from build123d import *

# Parameters (mm, degrees)
F0_W      = 95.881224
F0_H      = 68.022564
F0_R      = 16.769473
F1_DEPTH  = 25.4
F2_DEPTH  = 50.8
F4_DEPTH  = 25.4
F6_DEPTH  = 25.4
F8_DEPTH  = 0.254
F10_DEPTH = 0.0254


with BuildPart() as f1:
    # F0 (on Top) → F1 (new body)
    with BuildSketch(Plane.XY):
        Rectangle(F0_W, F0_H)
        Circle(F0_R, mode=Mode.SUBTRACT)
    extrude(amount=F1_DEPTH)

    # F0 (on Top) → F2 (join)
    with BuildSketch(Plane.XY):
        Circle(F0_R)
    extrude(amount=F2_DEPTH)

    # F3 (on Front) → F4 (cut)
    with BuildSketch(Plane.XZ):
        with BuildLine():
            ThreePointArc((16.7397, 50.897755), (-0.044019, 53.808078), (-16.71098, 50.290175))
            Line((-16.71098, 50.290175), (16.7397, 36.212575))
            Line((16.7397, 36.212575), (16.7397, 50.897755))
        make_face()
    extrude(amount=-F4_DEPTH, mode=Mode.SUBTRACT)

    # F5 (on Front) → F6 (cut)
    with BuildSketch(Plane.XZ):
        Polygon((-16.633531, 50.150838), (16.688788, 36.337622), (16.700679, 50.800726), (-16.633531, 50.828132), align=None)
    extrude(amount=F6_DEPTH, mode=Mode.SUBTRACT)

    # F7 (on Right) → F8 (cut)
    with BuildSketch(Plane.YZ):
        Polygon((-1.459569, 50.8672), (-1.681041, 36.348537), (0.976613, 36.348537), (0.976613, 50.8672), align=None)
    extrude(amount=F8_DEPTH, mode=Mode.SUBTRACT)

    # F9 (on Right) → F10 (cut)
    with BuildSketch(Plane.YZ):
        Polygon((-1.541382, 50.746284), (-1.648819, 36.371183), (0.972651, 36.371183), (0.972651, 50.746284), align=None)
    extrude(amount=-F10_DEPTH, mode=Mode.SUBTRACT)


solid = f1.part
Here's how the part is built. I have some questions about the finished solid (model axes, mm). A direction names the side the tool comes from. Round coordinates to 2 decimals unless told otherwise and drop trailing zeros. Loops run counter-clockwise (first coordinate to the right, second up) from the corner with the lowest first, then second, coordinate; pieces in that order, holes last. Notation, with made-up numbers: (33.25, 42) -> (67.25, 42) arc R7 cw to (67.25, 50) -> close; hole circle Ø4 at (79.25, 32.5). An arc over 180 degrees is marked (long way). Write each question's results on one line, items separated by ' | '.
(1) If we section it at C-C, the plane x = -26: List the corners of the cut face in (y, z) for me, then the cut area to 3 significant figures.
Worked answers:
outline: (-34.01, 0) -> (34.01, 0) -> (34.01, 25.4) -> (-34.01, 25.4) -> close | area: 1,730 mm2
(2) If we section it at A-A, the plane y = 5: List the corners of the cut face in (x, z) for me.
Worked answers:
outline: (-47.94, 0) -> (47.94, 0) -> (47.94, 25.4) -> (16.01, 25.4) -> (16.01, 36.52) -> (-16.01, 49.99) -> (-16.01, 25.4) -> (-47.94, 25.4) -> close; (-16.01, 50.58) arc R45.13 cw to (-15.44, 50.8) -> (-16.01, 50.8) -> close
(3) If we section it at B-B, the plane y = 21: List the corners of the cut face in (x, z) for me, then the cut area to 3 significant figures.
Worked answers:
outline: (-47.94, 0) -> (47.94, 0) -> (47.94, 25.4) -> (-47.94, 25.4) -> close | area: 2,440 mm2
(4) For faces 1 (the face through (-16.753, 0.737, 35.1)), 2 (the face through (-1, 0, 0)), 3 (the face through (-0.206, -6.404, 43.341)), which set-ups out of +Z, -Z, +X, -X, +Y, -Y let a thin tool reach every point of the face, with its end or its side?
Worked answers:
face 1: +Z | face 2: -Z, +X, -X, +Y, -Y | face 3: +Z, -Y
(5) For P1, Ø3, axis at y = -0.5, z = 40.5, coming from the +X side; P2, Ø0.5, axis at x = -16, z = 50.5, coming from the -Y side; P3, Ø20.5, axis at x = -3.5, y = 12.5, coming from the +Z side, each with a flat end and sliding along its axis, tell me the tip position at first contact or that it passes through.
Worked answers:
P1: x = 16.77 | P2: y = 0 | P3: z = 48.92
(6) We'd pull the mould along X, two halves only. Please class faces 4 (the face through (-11, 16, 25.4)), 5 (the face through (-0.22, 6.4, 43.35)), 6 (the face through (-47.941, 0, 13)), 7 (the face through (0.254, 0, 40)): released by +X, released by -X, zero draft, split by the parting line, or undercut.
Worked answers:
face 4: zero draft | face 5: undercut | face 6: released by -X | face 7: undercut
(7) If we section it at D-D, the plane z = 32.5: List the corners of the cut face in (x, y) for me, then the cut area to 3 significant figures.
Worked answers:
outline: circle Ø33.54 at (0, 0) | area: 883 mm2
(8) If I drill on L1, parallel to Z at x = 34, y = -30.5; L2, parallel to Z at x = -7.5, y = 0; L3, parallel to X at y = -3, z = 26, over which ranges is the centre line in solid material (lowest first)?
Worked answers:
L1: 0 to 25.4 | L2: 0 to 46.36 | L3: -16.5 to 16.5
